```python
from build123d import *

# Parameters (mm, degrees)
F0_W        = 52.1
F0_H        = 16
F1_DEPTH    = 5
F2_W        = 2
F2_H        = 16
F3_DEPTH    = 16
F4_W        = 6.5
F4_H        = 5.3
F5_DEPTH    = 195
F6_SIZE     = 1.5
F7_T1_DEPTH = 6.5
F8_DEPTH    = 3


# Not quite as in the source:
# - a fillet or chamfer that OpenCascade refuses, or shapes differently, is made with other operations: its cross-section is extruded or revolved along the edge and cut away or added


with BuildPart() as f1:
    # F0 (on Top) → F1 (new body)
    with BuildSketch(Plane.XY):
        with Locations((26.05, -8)):
            Rectangle(F0_W, F0_H)
    extrude(amount=F1_DEPTH)

    # F2 (on Top) → F3 (join)
    with BuildSketch(Plane.XY):
        with Locations((-1, -8)):
            Rectangle(F2_W, F2_H)
        with Locations((53.1, -8)):
            Rectangle(F2_W, F2_H)
    extrude(amount=F3_DEPTH)

    # F4 (on face) → F5 (cut, symmetric)
    with BuildSketch(Plane(origin=(52.1, 0, 0), x_dir=(0, -1, 0), z_dir=(-1, 0, 0))):
        with Locations((8, 10.65)):
            Rectangle(F4_W, F4_H)
    extrude(amount=F5_DEPTH, both=True, mode=Mode.SUBTRACT)

    # F6
    f6_edges = [f1.edges().sort_by_distance(p)[0] for p in [
        (52.1, -8, 16),
        (0, -8, 16),
    ]]
    chamfer(f6_edges, length=F6_SIZE)

    # F7: chamfer of 2.5 on 2 edges, made by hand

    # F7_s2 → F7_t1 (cut)
    with BuildSketch(Plane.XZ.offset(4.75)):
        Polygon((52.1, 15.8), (54.6, 13.3), (52.1, 13.3), align=None)
        Polygon((0, 15.8), (-2.5, 13.3), (0, 13.3), align=None)
    extrude(amount=F7_T1_DEPTH, mode=Mode.SUBTRACT)

    # F8 (cut): a face of the model
    f8_faces = [f1.faces().sort_by_distance(p)[0] for p in [
        (26.05, -8, 0),
    ]]
    extrude(f8_faces, amount=-F8_DEPTH, mode=Mode.SUBTRACT)


solid = f1.part
```
Model file for the job. Use its own axes, mm. A direction names the side the tool comes from. Give positions to 0.01 mm unless a question says otherwise; leave off trailing zeros. Loops run counter-clockwise (first coordinate to the right, second up) from the corner with the lowest first, then second, coordinate; pieces in that order, holes last. Notation, with made-up numbers: (1.25, 47) -> (14.25, 47) arc R31 ccw to (14.25, 78) -> close; hole circle Ø11 at (-12.75, 35.5). An arc over 180 degrees is marked (long way). Use CSV: the item, a comma, the result in double quotes. Start each with the question number.
1) Tool access for faces 5 (the flat face through (26, -8, 3)), 6 (the flat face through (52.1, -8.1, 7.6)), 7 (the flat face through (53, -8, 8)), 8 (the flat face through (-1, -11.25, 12)): list every direction of +Z, -Z, +X, -X, +Y, -Y with a clear straight run to the whole face (end or side of a thin tool).
2) Slice it at B-B on z = 9. Give the cut face in (x, y).
3) Slice it at A-A on z = 5.5. Give the cut face in (x, y).
4) Wall check: line 1 (X direction, y = -9.25, z = 6.25); line 2 (Z direction, x = 2, y = -9); line 3 (X direction, y = -9, z = 15.5). Give the ranges that are in metal, low to high.
5) Slice it at D-D on y = -12.25. Give the cut face in (x, z), plus the area to 3 significant figures.
6) Slice it at C-C on y = -6.75. Give the cut face in (x, z).
7) Mould opens along Y. For faces 1 (the flat face through (25.9, 0, 4.7)), 2 (the flat face through (0, -8.1, 7.6)), 3 (the flat face through (25.9, -16, 4.7)), 4 (the flat face through (53, -11.25, 12)) say: released by +Y, released by -Y, zero draft, split by the parting line, or undercut.
8) Flat gauge pins, fed straight in: pin 1 Ø8 at (x, y) = (28, -5.5) entering from +Z; pin 2 Ø1.5 at (x, z) = (37, 6.5) entering from +Y. Where does each tip first touch, or does it go through?
Computed values:
1,face 5,"-Z, +X, -X, +Y, -Y"
1,face 6,"+Z, +Y, -Y"
1,face 7,"+X, -X"
1,face 8,"none"
2,outline,"(-2, -16) -> (0, -16) -> (0, -11.25) -> (-2, -11.25) -> close; (-2, -4.75) -> (0, -4.75) -> (0, 0) -> (-2, 0) -> close; (52.1, -16) -> (54.1, -16) -> (54.1, -11.25) -> (52.1, -11.25) -> close; (52.1, -4.75) -> (54.1, -4.75) -> (54.1, 0) -> (52.1, 0) -> close"
3,outline,"(-2, -16) -> (0, -16) -> (0, 0) -> (-2, 0) -> close; (52.1, -16) -> (54.1, -16) -> (54.1, 0) -> (52.1, 0) -> close"
4,line 1,"x = -2 to 0, 52.1 to 54.1"
4,line 2,"z = 3 to 5"
4,line 3,"x = -2 to -1, 53.1 to 54.1"
5,outline,"(-2, 3) -> (54.1, 3) -> (54.1, 16) -> (53.6, 16) -> (52.1, 14.5) -> (52.1, 5) -> (0, 5) -> (0, 14.5) -> (-1.5, 16) -> (-2, 16) -> close"
5,area,"154 mm^2"
6,outline,"(-2, 3) -> (54.1, 3) -> (54.1, 8) -> (52.1, 8) -> (52.1, 5) -> (0, 5) -> (0, 8) -> (-2, 8) -> close; (-2, 13.8) -> (-0.65, 15.15) -> (-1.5, 16) -> (-2, 16) -> close; (52.75, 15.15) -> (54.1, 13.8) -> (54.1, 16) -> (53.6, 16) -> close"
7,face 1,"released by +Y"
7,face 2,"zero draft"
7,face 3,"released by -Y"
7,face 4,"undercut"
8,pin 1,"stops at z = 5"
8,pin 2,"passes through"
